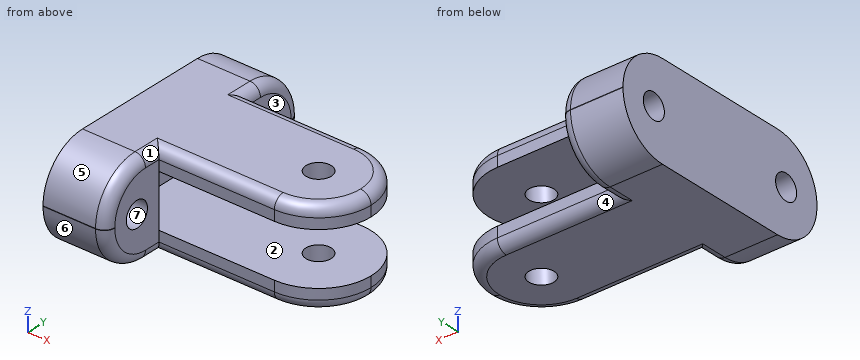
from build123d import *

# Parameters (mm, degrees)
SKETCH1_W             = 14.2875
SKETCH1_H             = 15.875
BOSS_EXTRUDE1_DEPTH   = 34.925
SKETCH2_W             = 7.9502
SKETCH2_H             = 15.875
CUT_EXTRUDE1_DEPTH    = 31.75
F_6_CLEARANCE_HOLE1_D = 3.7973
SKETCH5_W             = 14.2875
SKETCH5_H             = 9.525
BOSS_EXTRUDE2_DEPTH   = 9.525
F_6_CLEARANCE_HOLE2_D = 3.7973
FILLET1_R             = 7.112
FILLET3_R             = 7.9375
FILLET2_R             = 1.5875


with BuildPart() as part:
    # Sketch1 → Boss-Extrude1 (new body)
    with BuildSketch(Plane(origin=(0, 0, 0), x_dir=(0, 0, -1), z_dir=(1, 0, 0))):
        with Locations((7.14375, 7.9375)):
            Rectangle(SKETCH1_W, SKETCH1_H)
    extrude(amount=BOSS_EXTRUDE1_DEPTH)

    # Sketch2 → Cut-Extrude1 (cut)
    with BuildSketch(Plane(origin=(34.925, 0, 0), x_dir=(0, 0, -1), z_dir=(1, 0, 0))):
        with Locations((7.14375, 7.9375)):
            Rectangle(SKETCH2_W, SKETCH2_H)
    extrude(amount=-CUT_EXTRUDE1_DEPTH, mode=Mode.SUBTRACT)

    # #6 Clearance Hole1 (through all)
    with Locations(Plane(origin=(0, 0, -14.2875), x_dir=(-1, 0, 0), z_dir=(0, 0, -1))):
        with Locations((-27.0002, 7.9375)):
            Hole(F_6_CLEARANCE_HOLE1_D / 2)

    # Sketch5 → Boss-Extrude2 (add)
    with BuildSketch(Plane.ZY):
        with Locations((-7.14375, 20.6375)):
            Rectangle(SKETCH5_W, SKETCH5_H)
        with Locations((-7.14375, -4.7625)):
            Rectangle(SKETCH5_W, SKETCH5_H)
    extrude(amount=-BOSS_EXTRUDE2_DEPTH)

    # #6 Clearance Hole2 (through all)
    with Locations(Plane.ZY):
        with Locations((-7.14375, 19.84375), (-7.14375, -3.96875)):
            Hole(F_6_CLEARANCE_HOLE2_D / 2)

    # Fillet1
    fillet1_edges = [part.edges().sort_by_distance(p)[0] for p in [
        (4.7625, 25.4, -14.2875),
        (4.7625, 25.4, 0),
        (4.7625, -9.525, -14.2875),
        (4.7625, -9.525, 0),
    ]]
    fillet(fillet1_edges, radius=FILLET1_R)

    # Fillet3
    fillet3_edges = [part.edges().sort_by_distance(p)[0] for p in [
        (34.925, 0, -1.584325),
        (34.925, 0, -12.703175),
        (34.925, 15.875, -12.703175),
        (34.925, 15.875, -1.584325),
    ]]
    fillet(fillet3_edges, radius=FILLET3_R - 0.0001)  # a hair under: the kernel refuses the full size

    # Fillet2
    fillet2_edges = [part.edges().sort_by_distance(p)[0] for p in [
        (18.2563, 0, 0),
        (18.2563, 15.875, 0),
        (32.600189365, 13.550189365, 0),
        (32.600189365, 2.324810635, 0),
        (18.2563, 15.875, -14.2875),
        (18.2563, 0, -14.2875),
        (32.600189365, 13.550189365, -14.2875),
        (32.600189365, 2.324810635, -14.2875),
        (9.525, 17.0815, 0),
        (9.525, -1.2065, -14.2875),
        (9.525, 17.0815, -14.2875),
        (9.525, -9.525, -7.14375),
        (9.525, -1.2065, 0),
        (9.525, -7.441943428, -2.083056572),
        (9.525, -7.441943428, -12.204443428),
        (9.525, 25.4, -7.14375),
        (9.525, 23.316943428, -12.204443428),
        (9.525, 23.316943428, -2.083056572),
    ]]
    fillet(fillet2_edges, radius=FILLET2_R)


solid = part.part
The model under review builds one solid part; all positions refer to its coordinate system, in mm. Face numbers are marked on the shaded views. A direction names the side the tool comes from. Coordinates: 2 decimals unless noted, no trailing zeros. Loops run counter-clockwise (first coordinate to the right, second up) from the corner with the lowest first, then second, coordinate; pieces in that order, holes last.
(1) Insertion check: P1, Ø1.3, axis at x = 17.5, z = -2.5, coming from the +Y side (3 decimals); P2, Ø4, axis at y = 22, z = -9, coming from the +X side (3 decimals); P3, Ø0.5, axis at x = 21, z = -12.5, coming from the -Y side. Each pin has a flat end and moves straight along its axis. Give the tip position at first contact, or say it passes through.
Determined:
P1: stops at y = 15.875
P2: stops at x = 9.525
P3: stops at y = 0
(2) Draft analysis for pull direction Z (two halves, no side actions). For the marked faces 5, 6 and 7, state which applies: +Z half, -Z half, draft (parallel to the pull), parting line (faces both ways), or undercut.
Determined:
face 5: +Z half
face 6: -Z half
face 7: undercut
(3) Tool access review of the marked faces 1, 2, 3 and 4: name each direction out of +Z, -Z, +X, -X, +Y, -Y from which nothing blocks a thin tool from reaching the whole face with its end or side.
Determined:
face 1: +Z, +X, -Y
face 2: +X
face 3: +Z, -Z, +X, +Y
face 4: -Z, +X, +Y
(4) Consider section A-A, the plane x = 21.5. Give the boundary of the cut face in (y, z) (1 decimal), plus the area to 3 significant figures.
Determined:
outline: (0, -12.7) arc R1.6 ccw to (1.6, -14.3) - (14.3, -14.3) arc R1.6 ccw to (15.9, -12.7) - (15.9, -11.1) - (0, -11.1) - close; (0, -3.2) - (15.9, -3.2) - (15.9, -1.6) arc R1.6 ccw to (14.3, 0) - (1.6, 0) arc R1.6 ccw to (0, -1.6) - close
area: 98.4 mm2
(5) Wall thickness on L1, parallel to Z at x = 30, y = 11; L2, parallel to Y at x = 21.5, z = -11.5 (3 decimals); L3, parallel to Y at x = 2, z = -5.75: over which ranges is each line inside the solid? List them lowest first.
Determined:
L1: z = -14.29 to -11.12, -3.17 to 0
L2: y = 0 to 15.875
L3: y = -9.39 to -5.26, -2.68 to 18.55, 21.13 to 25.27
(6) Consider section B-B, the plane x = 6.5. Give the number of separate pieces and of enclosed holes in the cut face, plus the area to 3 significant figures.
Determined:
separate pieces: 1
enclosed holes: 3
area: 307 mm2
